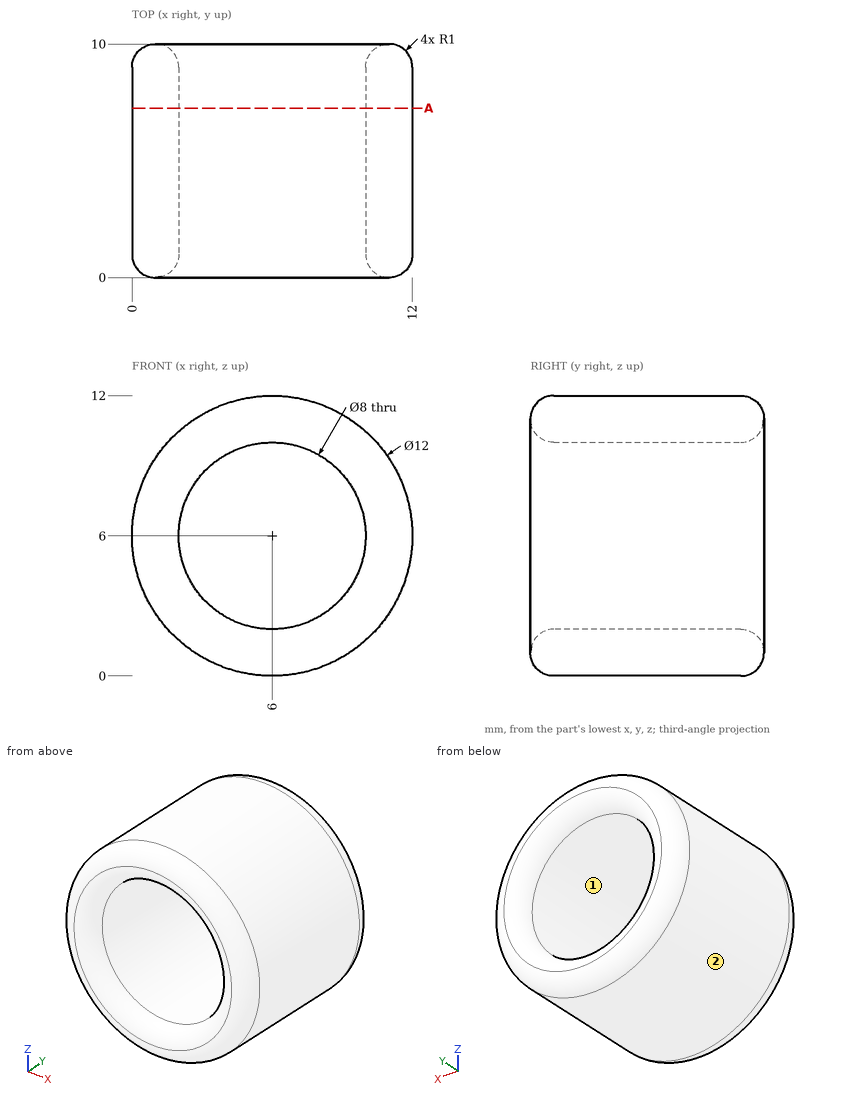
Can you work these out from the drawing? Everything is in mm from the part's minimum corner. Round coordinates to 2 decimals unless told otherwise and drop trailing zeros. Loops run counter-clockwise (first coordinate to the right, second up) from the corner with the lowest first, then second, coordinate; pieces in that order, holes last. Notation, with made-up numbers: (-16, 16) -> (12, 16) arc R4 ccw to (12, 23) -> close; hole circle Ø1 at (35.5, 40). An arc over 180 degrees is marked (long way). Put each result on its own line as item: value.
Q1. Thinking about a two-plate mould opening in Z: for the marked faces 1 and 2, which applies, pulls with the +Z half, pulls with the -Z half, needs draft (parallel to the pull), parting line crosses it, or undercut?
Checks:
face 1: undercut
face 2: parting line crosses it
Q2. I want a section at A-A on y = 7.25. Write out the boundary of the cut face in (x, z), and give its area (3 significant figures).
Checks:
outline: circle Ø12 at (6, 6); hole circle Ø8 at (6, 6)
area: 62.8 mm2
Q3. For pin 1 Ø1.5 at (x, y) = (5, 3.5) entering from +Z; pin 2 Ø3 at (x, y) = (10.5, 5) entering from +Z; pin 3 Ø1 at (y, z) = (1.5, 10) entering from -X, each with a flat end and sliding along its axis, tell me the tip position at first contact or that it passes through.
Checks:
pin 1: z = 11.99
pin 2: z = 11.2
pin 3: x = 1.13
Q4. Please list where these lines run through material, in increasing order: line 1 (X direction, y = 3.5, z = 6); line 2 (Z direction, x = 8.75, y = 1) (1 decimal); line 3 (Z direction, x = 6.25, y = 7.25) (3 decimals). Write a range as from..to.
Checks:
line 1: 0..2, 10..12
line 2: 0.7..3.1, 8.9..11.3
line 3: 0.005..2.008, 9.992..11.995
